```python
from build123d import *

# Parameters (mm, degrees)
SKETCH1_R           = 14.2875
BOSS_EXTRUDE1_DEPTH = 3.175
SKETCH2_R           = 9.525
SKETCH2_R_2         = 6.35
BOSS_EXTRUDE2_DEPTH = 12.7


with BuildPart() as part:
    # Sketch1 → Boss-Extrude1 (new body)
    with BuildSketch(Plane(origin=(0, 0, 0), x_dir=(1, 0, 0), z_dir=(0, 1, 0))):
        with Locations(Location((0, 0, 0), (0, 0, 270))):
            Circle(SKETCH1_R)
    extrude(amount=BOSS_EXTRUDE1_DEPTH)

    # Sketch2 → Boss-Extrude2 (add)
    with BuildSketch(Plane(origin=(0, 3.175, 0), x_dir=(1, 0, 0), z_dir=(0, 1, 0))):
        with Locations(Location((0, 0, 0), (0, 0, 270))):
            Circle(SKETCH2_R)
        with Locations(Location((0, 0, 0), (0, 0, 270))):
            Circle(SKETCH2_R_2, mode=Mode.SUBTRACT)
    extrude(amount=BOSS_EXTRUDE2_DEPTH)


solid = part.part
```
Geometry check sheet. Reference: the model listing, model coordinates, mm. A direction names the side the tool comes from. Coordinates: 2 decimals unless noted, no trailing zeros. Order: outer loops, then holes, each group sorted by start corner. A loop starts at its lowest first (then second) coordinate and runs counter-clockwise, first axis right, second up.
Item 1: Depth check by flat-ended pin: pin 1 (5 mm diameter, centred on x = -4.5, y = 13.5, fed in from +Z); pin 2 (1.5 mm diameter, centred on y = 12, z = 0, fed in from +X) (3 decimals); pin 3 (7.5 mm diameter, centred on x = 0, z = 0, fed in from +Y) (3 decimals). Enter the tip coordinate at first touch or a pass-through.
Item 2: Mould release check, pull along Z, two halves, no side actions. Record for faces 3 (the flat face through (0, 0, 0)), 4 (the cylindrical face through (0.628, 1.565, -14.274)), 5 (the flat face through (0, 3.175, 0)): released by +Z, released by -Z, zero draft, split by the parting line, or undercut.
Item 3: Tool access check on faces 1 (the flat face through (-6.2, 15.875, 2)), 2 (the cylindrical face through (-5.796, 9.436, -7.559)). Record the directions out of +Z, -Z, +X, -X, +Y, -Y that give a thin tool (end or side, any length) a straight path to the whole face; none if there is none.
Item 4: Section check D-D (x = 9). Enter the section's corners in (y, z) (3 decimals).
Item 5: Section check C-C (y = 8). Enter the section's corners in (x, z) (3 decimals), plus the area to 3 significant figures.
Item 6: Scan lines: line 1 along X through (y, z) = (7, 0) (3 decimals); line 2 along Y through (x, z) = (1.75, -4.5) (3 decimals); line 3 along Z through (x, y) = (-4.5, 9.75). Record each from-to range of solid material in increasing order.
Check sheet entries:
1. pin 1: stops at z = 9.31
1. pin 2: stops at x = 9.525
1. pin 3: stops at y = 3.175
2. face 3: zero draft
2. face 4: split by the parting line
2. face 5: undercut
3. face 1: +Z, -Z, +X, -X, +Y
3. face 2: +Y
4. outline: (0, -11.097) - (3.175, -11.097) - (3.175, -3.119) - (15.875, -3.119) - (15.875, 3.119) - (3.175, 3.119) - (3.175, 11.097) - (0, 11.097) - close
5. outline: circle Ø19.05 at (0, 0); hole circle Ø12.7 at (0, 0)
5. area: 158 mm2
6. line 1: x = -9.525 to -6.35, 6.35 to 9.525
6. line 2: y = 0 to 3.175
6. line 3: z = -8.39 to -4.48, 4.48 to 8.39
